from build123d import *

# Parameters (mm, degrees)
F1_DEPTH = 15
F3_DEPTH = 45.6627906977
F4_R     = 3.5
F5_DEPTH = 3.8400468949
F6_W     = 45.6627906977
F6_H     = 31.9253331743
F6_R     = 3.5
F6_R_2   = 1.5
F7_DEPTH = 1


with BuildPart() as f1:
    # F0 (on Front) → F1 (new body)
    with BuildSketch(Plane.XZ):
        Polygon((19.25, 0), (-19.25, 0), (-19.25, 21.5), (-12.5, 21.5), (-12.5, 23.5), (-22.8313953488, 23.5), (-22.8313953488, -2), (22.8313953488, -2), (22.8313953488, 23.5), (12.5, 23.5), (12.5, 21.5), (19.25, 21.5), align=None)
    extrude(amount=F1_DEPTH)

    # F2 (on face) → F3 (join, through all)
    with BuildSketch(Plane.YZ.offset(22.8313953488)):
        Polygon((0, -2), (-30, -2), (0, -12.919107028), align=None)
    extrude(amount=-F3_DEPTH)

    # F4 (on face) → F5 (cut, through all)
    with BuildSketch(Plane(origin=(0, -4.1521209629, -11.4078585884), x_dir=(1, 0, 0), z_dir=(0, -0.3420201433, -0.9396926208))):
        with Locations((0, 20.459043681)):
            Circle(F4_R)
    extrude(amount=-F5_DEPTH, mode=Mode.SUBTRACT)

    # F6 (on face) → F7 (join)
    with BuildSketch(Plane(origin=(0, -4.1521209629, -11.4078585884), x_dir=(1, 0, 0), z_dir=(0, -0.3420201433, -0.9396926208))):
        with Locations((0, 11.5440717498)):
            Rectangle(F6_W, F6_H)
        with Locations((0, 20.459043681)):
            Circle(F6_R, mode=Mode.SUBTRACT)
        with Locations((0, 20.459043681)):
            Circle(F6_R)
        with Locations((0, 20.459043681)):
            Circle(F6_R_2, mode=Mode.SUBTRACT)
    extrude(amount=F7_DEPTH)


solid = f1.part
Read the model definition and answer for the solid it produces. Units are mm, in the model's axes. A direction names the side the tool comes from. Round coordinates to 2 decimals unless told otherwise and drop trailing zeros. Write each loop counter-clockwise with the first axis right and the second up, starting at its lowest first coordinate (ties: lowest second). Pieces come first, ordered by that corner, then holes. Notation, with made-up numbers: (-12, 35.25) - (19, 35.25) arc R19 ccw to (19, 69.25) - close; hole circle Ø11 at (82.5, -6.5). An arc over 180 degrees is marked (long way). One line per question, with ' | ' between items. Start each with the question number.
1. Section C-C (x = 9.5) is taken. Determine the outline of the cut face in (y, z).
2. Section B-B (x = -15) is taken. Determine the outline of the cut face in (y, z).
3. For faces 1 (the face through (-16, -7, 21.5)), 2 (the face through (12.5, -7, 23)), 3 (the face through (1.51, -22.69, -4.66)), 4 (the face through (0, -15, -1)), determine the directions among +Z, -Z, +X, -X, +Y, -Y from which every point of the face is accessible in a straight line to the end or side of a thin tool.
4. Each of these flat-tipped pins is pushed along its axis until it touches: pin 1 (3 mm diameter, centred on x = 6.5, y = -17, fed in from -Z); pin 2 (8 mm diameter, centred on x = -6.5, y = -25.5, fed in from -Z); pin 3 (7.5 mm diameter, centred on x = -2, z = 6, fed in from -Y); pin 4 (4.5 mm diameter, centred on x = 6.5, y = -7.5, fed in from +Z). Where does it stop, or does it pass through?
5. Find the intervals of material crossed by probe 1 along X at (y, z) = (-3, 3); probe 2 along Y at (x, z) = (19.5, 4); probe 3 along Z at (x, y) = (10, -12), in increasing order. Write a range as [from, to].
6. For a pull along X with two mould halves and no side action, classify faces 5 (the face through (22.831, -7, 3)), 6 (the face through (0, -27, -2)), 7 (the face through (-0.759, -19.665, -4.201)) as +X half, -X half, draft (parallel to the pull), parting line (faces both ways), or undercut.
7. Section A-A (z = 18.5) is taken. Determine the outline of the cut face in (x, y).
8. Section D-D (y = -6.5) is taken. Determine the outline of the cut face in (x, z).
Filled in:
1) outline: (-30.34, -2.94) - (-0.34, -13.86) - (0, -12.92) - (0, 0) - (-15, 0) - (-15, -2) - (-30, -2) - close
2) outline: (-30.34, -2.94) - (-0.34, -13.86) - (0, -12.92) - (0, 0) - (-15, 0) - (-15, -2) - (-30, -2) - close; (-15, 21.5) - (0, 21.5) - (0, 23.5) - (-15, 23.5) - close
3) face 1: +Y, -Y | face 2: +Z, +Y, -Y | face 3: none | face 4: +Z, +X, -X, -Y
4) pin 1: z = -8.34 | pin 2: z = -6.16 | pin 3: through | pin 4: z = 0
5) probe 1: [-22.83, -19.25], [19.25, 22.83] | probe 2: [-15, 0] | probe 3: [-9.62, 0]
6) face 5: +X half | face 6: draft | face 7: undercut
7) outline: (-22.83, -15) - (-19.25, -15) - (-19.25, 0) - (-22.83, 0) - close; (19.25, -15) - (22.83, -15) - (22.83, 0) - (19.25, 0) - close
8) outline: (-22.83, -11.62) - (22.83, -11.62) - (22.83, 23.5) - (12.5, 23.5) - (12.5, 21.5) - (19.25, 21.5) - (19.25, 0) - (-19.25, 0) - (-19.25, 21.5) - (-12.5, 21.5) - (-12.5, 23.5) - (-22.83, 23.5) - close
